from build123d import *

# Parameters (mm, degrees)
F1_DEPTH = 3.81
F2_DEPTH = 25.4


with BuildPart() as f1:
    # F0 (on Top) → F1 (new body)
    with BuildSketch(Plane.XY):
        Polygon((6.5642443103, 3.7926732977), (-0.0024292689, 7.5811389783), (-6.5666735793, 3.7884656805), (-6.5642443103, -3.7926732977), (0.0024292689, -7.5811389783), (6.5666735793, -3.7884656805), align=None)
        Polygon((-4.0262038002, 2.3228099792), (-0.00148945, 4.6481997614), (4.0247143502, 2.3253897822), (4.0262038002, -2.3228099792), (0.00148945, -4.6481997614), (-4.0247143502, -2.3253897822), align=None, mode=Mode.SUBTRACT)
    extrude(amount=F1_DEPTH)

    # F2 (add): a face of the model
    f2_faces = [f1.faces().sort_by_distance(p)[0] for p in [
        (6.5654589448, 0.0021038086, 1.905),
    ]]
    extrude(f2_faces, amount=F2_DEPTH)


solid = f1.part
Verification items for the finished model (mm, model axes). A direction names the side the tool comes from. Coordinates: 2 decimals unless noted, no trailing zeros. Order: outer loops, then holes, each group sorted by start corner. A loop starts at its lowest first (then second) coordinate and runs counter-clockwise, first axis right, second up. Notation, with made-up numbers: M -22,79 L 19,79 A17 cw 19,100 Z; hole C -12,75 d1. An arc over 180 degrees is marked long. Return JSON: item names as keys, results as strings.
1) Access from +Z, -Z, +X, -X, +Y, -Y to the whole of each face (thin tool, end or side, straight path). Record for faces 5 (the flat face through (2.04, -3.47, 1.88)), 6 (the flat face through (12, 0, 0)).
Answer list:
{"face 5": "+Z, -Z", "face 6": "-Z, +X, -X, +Y, -Y"}
2) Thickness scan on L1, parallel to X at y = -1.5, z = 2.7; L2, parallel to Y at x = 29, z = 2.75; L3, parallel to Y at x = -0.5, z = 2.15. Record the ranges inside material, lowest first. Write a range as [from, to].
Answer list:
{"L1": "[-6.56, -4.02], [4.03, 31.97]", "L2": "[-3.78, 3.8]", "L3": "[-7.29, -4.36], [4.36, 7.29]"}
3) Cross-section at A-A, the plane z = 2.7. Record the boundary of the cut face in (x, y).
Answer list:
{"outline": "M -6.57,3.79 L -6.56,-3.79 L 0,-7.58 L 6.57,-3.79 L 31.97,-3.78 L 31.96,3.8 L 6.56,3.79 L 0,7.58 Z; hole M -4.03,2.32 L -4.02,-2.33 L 0,-4.65 L 4.03,-2.32 L 4.02,2.33 L 0,4.65 Z"}
4) Cross-section at D-D, the plane x = 29. Record the boundary of the cut face in (y, z).
Answer list:
{"outline": "M -3.78,0 L 3.8,0 L 3.8,3.81 L -3.78,3.81 Z"}
5) Release check for a two-part mould opening along X. For faces 1 (the flat face through (-1.983, -3.503, 1.878)), 2 (the flat face through (3.24, -5.71, 1.88)), 3 (the flat face through (-3.33, -5.66, 1.88)), 4 (the flat face through (-2.04, 3.47, 1.88)) record: +X half, -X half, draft (parallel to the pull), parting line (faces both ways), or undercut.
Answer list:
{"face 1": "undercut", "face 2": "+X half", "face 3": "-X half", "face 4": "undercut"}
6) Cross-section at B-B, the plane x = 1. Record the boundary of the cut face in (y, z), and give its area (3 significant figures).
Answer list:
{"outline": "M -7,0 L -4.07,0 L -4.07,3.81 L -7,3.81 Z; M 4.07,0 L 7,0 L 7,3.81 L 4.07,3.81 Z", "area": "22.3 mm2"}
7) Cross-section at C-C, the plane y = 0. Record the boundary of the cut face in (x, z), and give its area (3 significant figures).
Answer list:
{"outline": "M -6.57,0 L -4.03,0 L -4.03,3.81 L -6.57,3.81 Z; M 4.03,0 L 31.97,0 L 31.97,3.81 L 4.03,3.81 Z", "area": "116 mm2"}
8) Gauge pin test, flat ends, axial feed: pin 1 (2 mm diameter, centred on x = 10.5, z = 2, fed in from -Y); pin 2 (2 mm diameter, centred on x = 12.5, z = 1.5, fed in from +Y). Record the tip position at first contact, or that the pin passes through.
Answer list:
{"pin 1": "y = -3.79", "pin 2": "y = 3.79"}
